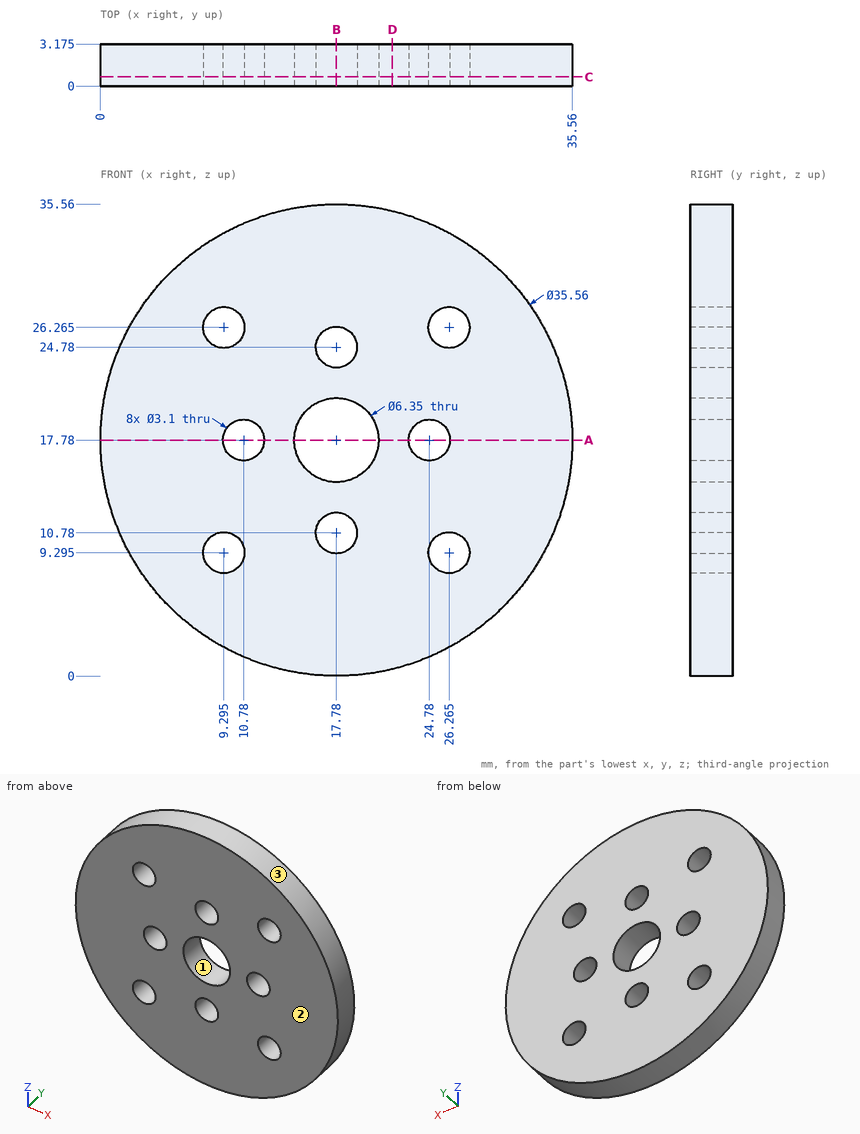
Job drawing, mm, ordinate dimensions from the low corner. One solid piece. Coordinates: 2 decimals unless noted, no trailing zeros. Loops run counter-clockwise (first coordinate to the right, second up) from the corner with the lowest first, then second, coordinate; pieces in that order, holes last. Notation, with made-up numbers: (22.25, -4) -> (76.25, -4) arc R21 ccw to (76.25, 14) -> close; hole circle Ø8 at (-9.75, -33). An arc over 180 degrees is marked (long way). One line per item, written item: value.
1. Slice it at C-C on y = 0.7. Give the number of separate pieces and of enclosed holes in the cut face, and give its area (3 significant figures).
Answers:
separate pieces: 1
enclosed holes: 9
area: 901 mm^2
2. Slice it at B-B on x = 17.78. Write the cut outline in (y, z) (1 decimal).
Answers:
outline: (0, 0) -> (3.2, 0) -> (3.2, 9.2) -> (0, 9.2) -> close; (0, 12.3) -> (3.2, 12.3) -> (3.2, 14.6) -> (0, 14.6) -> close; (0, 21) -> (3.2, 21) -> (3.2, 23.2) -> (0, 23.2) -> close; (0, 26.3) -> (3.2, 26.3) -> (3.2, 35.6) -> (0, 35.6) -> close
3. Pull direction X, two halves, no side cores. Call the marked faces 1, 2 and 3: pulls with the +X half, pulls with the -X half, needs draft (parallel to the pull), parting line crosses it, or undercut.
Answers:
face 1: undercut
face 2: needs draft
face 3: parting line crosses it
4. Slice it at D-D on x = 22. Write the cut outline in (y, z) (1 decimal).
Answers:
outline: (0, 0.5) -> (3.2, 0.5) -> (3.2, 35.1) -> (0, 35.1) -> close
5. Drill centre lines: line 1 (X direction, y = 1.85, z = 17.78) (1 decimal); line 2 (X direction, y = 1.35, z = 8) (1 decimal); line 3 (X direction, y = 2.55, z = 9.5) (1 decimal). Where is each one in solid material? Low to high. Write a range as [from, to].
Answers:
line 1: x = [0, 9.2], [12.3, 14.6], [21, 23.2], [26.3, 35.6]
line 2: x = [2.9, 8.4], [10.1, 25.4], [27.1, 32.6]
line 3: x = [2, 7.8], [10.8, 16.9], [18.7, 24.7], [27.8, 33.5]
6. Slice it at A-A on z = 17.78. Write the cut outline in (x, y) (1 decimal).
Answers:
outline: (0, 0) -> (9.2, 0) -> (9.2, 3.2) -> (0, 3.2) -> close; (12.3, 0) -> (14.6, 0) -> (14.6, 3.2) -> (12.3, 3.2) -> close; (21, 0) -> (23.2, 0) -> (23.2, 3.2) -> (21, 3.2) -> close; (26.3, 0) -> (35.6, 0) -> (35.6, 3.2) -> (26.3, 3.2) -> close
